Autodesk Inventor part; units mm, degrees
ref_plane "Plano de trabajo1" through (39.4603, 28.9326, 43.4345) normal (-0.0230448, -0.9802565, 0.1963824) x (0.9993754, -0.0278517, -0.0217506)
ref_plane "YZ Plane" through (0, 0, 0) normal (1, 0, 0) x (0, 1, 0)
ref_plane "XZ Plane" through (0, 0, 0) normal (0, 1, 0) x (-1, 0, 0)
ref_plane "Plano de trabajo1" through (39.4603, 28.9326, 43.4345) normal (-0.0230448, -0.9802565, 0.1963824) x (0.9993754, -0.0278517, -0.0217506)
sketch "Boceto1" plane through (39.4603, 28.9326, 43.4345) normal (-0.0230448, -0.9802565, 0.1963824) x (0.9993754, -0.0278517, -0.0217506)
  circle A0 centre (25.7474, -0.0015) radius 6 construction
  circle A1 centre (25.7474, -0.0015) radius 8.5 construction
  circle A2 centre (25.7474, -0.0015) radius 8.5
  line L0 (73.7302, -52.0094) -> (-22.2354, -52.0094)
  line L1 (-22.2354, -52.0094) -> (-22.2354, 52.0063)
  line L2 (-22.2354, 52.0063) -> (73.7302, 52.0063)
  line L3 (73.7302, 52.0063) -> (73.7302, -52.0094)
  line L4 (73.7302, -52.0094) -> (-22.2354, 52.0063) construction
  line L5 (-22.2354, -52.0094) -> (73.7302, 52.0063) construction
  line L6 (18.0272, 52.0081) -> (-18.0728, 52.0046) construction
  line L7 (73.7311, 10.0133) -> (73.7292, 30.0133) construction
  circle A3 centre (11.587, -43.5711) radius 5.65 construction
  circle A4 centre (11.587, -43.5711) radius 5.65
  line L8 (77.9675, -50.0094) -> (77.9675, 50.0063)
  line L9 (73.7302, 52.0063) -> (77.9675, 52.0063)
  line L10 (77.9675, 52.0063) -> (77.9675, -52.0094)
  line L11 (77.9675, -52.0094) -> (73.7302, -52.0094)
  line L12 (73.7302, -52.0094) -> (73.7302, 52.0063)
  line L13 (77.9675, 17.0063) -> (74.9675, 17.0063)
  line L14 (77.9675, 37.0063) -> (74.9675, 37.0063)
  line L15 (77.9675, -37.0094) -> (74.9675, -37.0094)
  line L16 (77.9675, -17.0094) -> (74.9675, -17.0094)
  line L17 (77.9675, -37.0094) -> (73.7302, -37.0094)
  line L18 (73.7302, -37.0094) -> (73.7302, -17.0094)
  line L19 (73.7302, -17.0094) -> (77.9675, -17.0094)
  line L20 (77.9675, -17.0094) -> (77.9675, -37.0094)
  line L21 (77.9675, 17.0063) -> (73.7302, 17.0063)
  line L22 (73.7302, 17.0063) -> (73.7302, 37.0063)
  line L23 (73.7302, 37.0063) -> (77.9675, 37.0063)
  line L24 (77.9675, 37.0063) -> (77.9675, 17.0063)
  line L25 (77.9675, 52.0063) -> (80.9675, 52.0063)
  line L26 (80.9675, 52.0063) -> (80.9675, 37.0063)
  line L27 (80.9675, 37.0063) -> (77.9675, 37.0063)
  line L28 (77.9675, 37.0063) -> (77.9675, 52.0063)
  line L29 (77.9675, 17.0063) -> (80.9675, 17.0063)
  line L30 (80.9675, 17.0063) -> (80.9675, -17.0094)
  line L31 (80.9675, -17.0094) -> (77.9675, -17.0094)
  line L32 (77.9675, -17.0094) -> (77.9675, 17.0063)
  line L33 (77.9675, -37.0094) -> (80.9675, -37.0094)
  line L34 (80.9675, -37.0094) -> (80.9675, -52.0094)
  line L35 (80.9675, -52.0094) -> (77.9675, -52.0094)
  line L36 (77.9675, -52.0094) -> (77.9675, -37.0094)
  point P0 (-37.6851, -49.2992)
  point P1 (73.7302, 20.0133)
  point P2 (-0.0228, 52.0063)
  point P3 (77.9675, -0.0015)
  point P4 (76.4675, -17.0094)
  point P5 (77.9675, -50.0094)
  point P6 (74.9675, -37.0094)
  point P7 (74.9675, 17.0063)
  point P8 (73.7302, 17.0063)
  point P9 (73.7302, -17.0094)
  point P10 (74.9675, -17.0094)
  point P11 (73.7302, 37.0063)
  point P12 (74.9675, 37.0063)
  point P13 (77.9675, 50.0063)
  point P14 (77.9675, -52.0094)
  point P15 (77.9675, -17.0094)
  point P16 (77.9675, 37.0063)
  dimension "d33" = 3
extrude "Extrusión1" add sketch "Boceto1" along normal blind 3
sketch "Boceto3" plane through (39.3912, 25.9918, 44.0236) normal (-0.0230448, -0.9802565, 0.1963824) x (0.9993754, -0.0278517, -0.0217506)
  line L0 (44.9302, -50.0094) -> (44.9302, 50.0063) construction
  line L1 (47.9302, -50.0094) -> (47.9302, 50.0063) construction
  line L2 (44.9302, 37.0063) -> (47.9302, 37.0063)
  line L3 (47.9302, 37.0063) -> (47.9302, 17.0063)
  line L4 (47.9302, 17.0063) -> (44.9302, 17.0063)
  line L5 (44.9302, 17.0063) -> (44.9302, 37.0063)
  line L6 (73.7302, 52.0063) -> (-22.2354, 52.0063) construction
  line L7 (44.9302, -17.0094) -> (47.9302, -17.0094)
  line L8 (47.9302, -17.0094) -> (47.9302, -37.0094)
  line L9 (47.9302, -37.0094) -> (44.9302, -37.0094)
  line L10 (44.9302, -37.0094) -> (44.9302, -17.0094)
  line L11 (-22.2354, -52.0094) -> (73.7302, -52.0094) construction
  point P0 (-37.6851, -49.2992)
  point P1 (-22.2354, 52.0063)
  point P2 (-22.2354, -52.0094)
  point P3 (73.7302, -52.0094)
  point P4 (46.4302, -37.0094)
  dimension "d2" = 20
  dimension "d3" = 15
  dimension "d4" = 15
  dimension "d5" = 20
extrude "Extrusión2" [suppressed]
sketch "Boceto4" plane through (39.3912, 25.9918, 44.0236) normal (-0.0230448, -0.9802565, 0.1963824) x (0.9993754, -0.0278517, -0.0217506)
  circle A0 centre (62.9302, -47.0094) radius 1.6 construction
  circle A1 centre (62.9302, -37.0094) radius 1.6 construction
  circle A2 centre (62.9302, 37.0063) radius 1.6 construction
  circle A3 centre (62.9302, 47.0063) radius 1.6 construction
  point P0 (-37.6851, -49.2992)
hole "Agujero1" at (101.0227, 15.0366, -3.4278) at (101.2906, 16.9942, 6.3751) at (103.2735, 31.4834, 78.9317) at (103.5414, 33.441, 88.7345) direction (0.0230448, 0.9802565, -0.1963824) diameter 3 end through all
sketch "Boceto5" plane through (39.3912, 25.9918, 44.0236) normal (-0.0230448, -0.9802565, 0.1963824) x (0.9993754, -0.0278517, -0.0217506)
  line L0 (-22.2354, 52.0063) -> (-22.2354, -52.0094) construction
  line L1 (-22.2354, -52.0094) -> (73.7302, -52.0094) construction
  circle A0 centre (-10.3398, 19.9988) radius 1.6 construction
  circle A1 centre (-10.3398, -0.0012) radius 1.6 construction
  point P0 (-37.6851, -49.2992)
  point P1 (-2.2354, -0.0015)
  point P2 (-22.2354, -0.0015)
  dimension "d16" = 20
  dimension "d18" = 0
hole "Agujero2" at (37.1571, 26.0538, 44.0708) at (29.5936, 30.1947, 63.853) at (29.0578, 26.2796, 44.2473) direction (0.0230448, 0.9802565, -0.1963824) diameter 3 end through all
sketch "Boceto6" plane through (39.3912, 25.9918, 44.0236) normal (-0.0230448, -0.9802565, 0.1963824) x (0.9993754, -0.0278517, -0.0217506)
  line L0 (70.7302, 30.0063) -> (62.7302, 30.0063)
  line L1 (62.7302, 30.0063) -> (62.7302, 27.0063)
  line L2 (62.7302, 27.0063) -> (70.7302, 27.0063)
  line L3 (70.7302, 27.0063) -> (70.7302, 30.0063)
  line L4 (70.7302, 30.0063) -> (62.7302, 27.0063) construction
  line L5 (62.7302, 30.0063) -> (70.7302, 27.0063) construction
  line L6 (73.7302, 17.0063) -> (73.7302, 37.0063) construction
  line L7 (73.7302, 52.0063) -> (-22.2354, 52.0063) construction
  point P0 (-37.6851, -49.2992)
  point P1 (66.7302, 28.5063)
  point P2 (73.7302, -52.0094)
  point P3 (70.7302, 28.5063)
  dimension "d26" = 8
  dimension "d27" = 3
  dimension "d28" = 3
  dimension "d29" = 22
extrude "Extrusión3" cut sketch "Boceto6" against normal through all
fillet "Empalme1" radius 2 8 edges at (18.5975, 38.2622, 95.1938) (15.8108, 17.9002, -6.7714) (121.736, 35.3878, 92.9491) (121.3341, 32.4514, 78.2448) (120.7983, 28.5363, 58.6391) (119.887, 21.8774, 25.2939) (119.3512, 17.9622, 5.6882) (118.9493, 15.0258, -9.0161)
properties part number "BaseMotoJose"
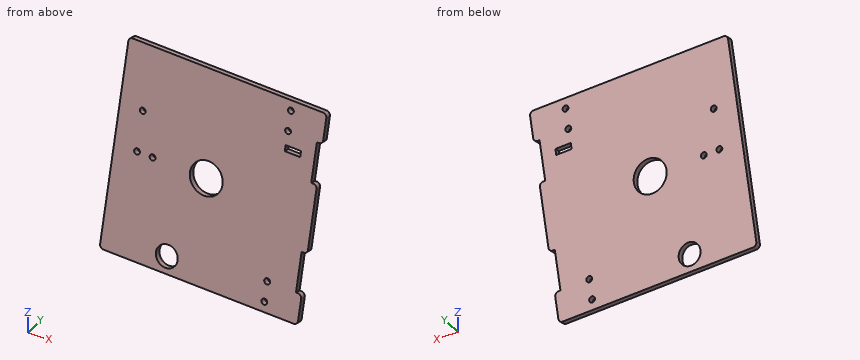
Verification items for the finished model (mm, model axes). Coordinates: 2 decimals unless noted, no trailing zeros. Loops run counter-clockwise (first coordinate to the right, second up) from the corner with the lowest first, then second, coordinate; pieces in that order, holes last. Notation, with made-up numbers: (-1, 50) -> (39, 50) arc R21 ccw to (39, 65) -> close; hole circle Ø6 at (14.25, -25). An arc over 180 degrees is marked (long way). Answer as a JSON object with one key per item and string values. Group by question number.
Item 1: Depth check by flat-ended pin: pin 1 (4 mm diameter, centred on x = 61.5, z = 54.5, fed in from -Y); pin 2 (4 mm diameter, centred on x = 110, y = 18, fed in from -Z); pin 3 (6 mm diameter, centred on x = 104, z = 66, fed in from +Y). Enter the tip coordinate at first touch or a pass-through.
Item 2: Sectioned sample at B-B on x = 86. Record the boundary of the cut face in (y, z).
Item 3: Sectioned sample at A-A on z = 10. Record the boundary of the cut face in (x, y).
Item 4: Scan lines: probe 1 along Y at (x, z) = (43.5, 67); probe 2 along Y at (x, z) = (22, 29.5). Record each from-to range of solid material in increasing order.
Evaluation:
{
 "1": {"pin 1": "stops at y = 27.17", "pin 2": "stops at z = -9.15", "pin 3": "stops at y = 32.52"},
 "2": {"outline": "(14.47, -8.01) -> (17.42, -8.59) -> (37.86, 93.43) -> (34.91, 94.02) -> close"},
 "3": {"outline": "(16.23, 19.72) -> (116.43, 17.36) -> (116.51, 20.42) -> (16.31, 22.78) -> close"},
 "4": {"probe 1": "y = 30.5 to 33.56", "probe 2": "y = 23.49 to 26.55"}
}
